```python
from build123d import *

# Parameters (mm, degrees)
SKETCH1_R           = 15
SKETCH1_R_2         = 14
BOSS_EXTRUDE1_DEPTH = 12
CUT_EXTRUDE1_DEPTH  = 31
CIRPATTERN1_COUNT   = 5
CUT_EXTRUDE2_DEPTH  = 32
CIRPATTERN2_COUNT   = 10


with BuildPart() as part:
    # Sketch1 → Boss-Extrude1 (new body)
    with BuildSketch(Plane.XY):
        Circle(SKETCH1_R)
        Circle(SKETCH1_R_2, mode=Mode.SUBTRACT)
    extrude(amount=BOSS_EXTRUDE1_DEPTH)

    # Sketch2 → Cut-Extrude1 (cut, symmetric)
    with BuildSketch(Plane(origin=(0, 0, 0), x_dir=(0, 0, -1), z_dir=(1, 0, 0))):
        Polygon((-1.5, 0), (-1.5, 3.5), (-10.5, 0), (-1.5, -3.5), align=None)
    cut_extrude1 = extrude(amount=CUT_EXTRUDE1_DEPTH, both=True, mode=Mode.SUBTRACT)

    # CirPattern1: Cut-Extrude1 ×5 about axis
    cirpattern1_axis = Axis((0, 0, 0), (0, 0, 1))
    for i in range(1, CIRPATTERN1_COUNT):
        add(cut_extrude1.rotate(cirpattern1_axis, i * 360 / CIRPATTERN1_COUNT), mode=Mode.SUBTRACT)

    # Sketch7 → Cut-Extrude2 (cut)
    with BuildSketch(Plane(origin=(-4.635254916, 14.265847744, 0), x_dir=(0.9510565162951501, 0.30901699437495833, 0), z_dir=(-0.30901699437495833, 0.9510565162951502, 0))):
        Polygon((-1.041848082, -10.5), (-4.541848082, -1.5), (-7.776778784, -10.5), align=None)
    cut_extrude2 = extrude(amount=-CUT_EXTRUDE2_DEPTH, mode=Mode.SUBTRACT)

    # CirPattern2: Cut-Extrude2 ×10 about axis
    cirpattern2_axis = Axis((0, 0, 0), (0, 0, 1))
    for i in range(1, CIRPATTERN2_COUNT):
        add(cut_extrude2.rotate(cirpattern2_axis, i * 360 / CIRPATTERN2_COUNT), mode=Mode.SUBTRACT)


solid = part.part
```
The model under review builds one solid part; all positions refer to its coordinate system, in mm. A direction names the side the tool comes from. Give positions to 0.01 mm unless a question says otherwise; leave off trailing zeros. Write each loop counter-clockwise with the first axis right and the second up, starting at its lowest first coordinate (ties: lowest second). Pieces come first, ordered by that corner, then holes. Notation, with made-up numbers: M 52,22 L 90,22 A18 ccw 90,42 Z; hole C 65,-24 d6. An arc over 180 degrees is marked long. Answer in a Markdown table with one row per item.
Item 1: Add section C-C on y = -2. Give the boundary of the cut face in (x, z), plus the area to 3 significant figures.
Check sheet entries:
| item | result |
|---|---|
| outline | M -14.87,0 L -13.86,0 L -13.86,1.5 L -14.87,1.5 Z; M -14.87,5.36 L -13.86,5.36 L -13.86,7.02 L -14.48,8.04 L -14.87,8.04 Z; M -14.87,10.5 L -13.86,10.5 L -13.86,12 L -14.87,12 Z; M 13.86,0 L 14.87,0 L 14.87,1.5 L 13.86,1.5 Z; M 13.86,5.36 L 14.87,5.36 L 14.87,8.04 L 14.48,8.04 L 13.86,7.02 Z; M 13.86,10.5 L 14.87,10.5 L 14.87,12 L 13.86,12 Z |
| area | 10.8 mm2 |
Item 2: Add section A-A on x = 7. Give the boundary of the cut face in (y, z).
Check sheet entries:
| item | result |
|---|---|
| outline | M -13.27,0 L -12.12,0 L -12.12,1.5 L -13.27,1.5 Z; M -13.27,3.92 L -12.12,3.02 L -12.12,4.71 L -12.8,6.23 L -13.27,6.6 Z; M -13.27,10.5 L -12.12,10.5 L -12.12,12 L -13.27,12 Z; M 12.12,0 L 13.27,0 L 13.27,1.5 L 12.12,1.5 Z; M 12.12,3.02 L 13.27,3.92 L 13.27,6.6 L 12.8,6.23 L 12.12,4.71 Z; M 12.12,10.5 L 13.27,10.5 L 13.27,12 L 12.12,12 Z |
Item 3: Add section B-B on z = 11. Give the boundary of the cut face in (x, y).
Check sheet entries:
| item | result |
|---|---|
| outline | C 0,0 d30; hole C 0,0 d28 |
Item 4: Add section D-D on z = 6.75. State how many separate pieces and enclosed holes the cut face has, plus the area to 3 significant figures.
Check sheet entries:
| item | result |
|---|---|
| separate pieces | 20 |
| enclosed holes | 0 |
| area | 18.7 mm2 |
Item 5: For P1, Ø1.6, axis at x = -9.5, y = -10.5, coming from the -Z side; P2, Ø1.5, axis at x = -4, z = 8.5, coming from the -Y side; P3, Ø4, axis at x = 7, z = 9.5, coming from the -Y side; P4, Ø5, axis at x = 5, z = 7, coming from the +Y side, all flat-tipped, find the tip position at first contact; note any pin that passes through.
Check sheet entries:
| item | result |
|---|---|
| P1 | z = 0 |
| P2 | y = -14.64 |
| P3 | y = -14.14 |
| P4 | y = 14.79 |
Item 6: Draft analysis for pull direction X (two halves, no side actions). For faces 3 (the face through (-10.164, 10.805, 6.063)), 4 (the face through (-6.1, 13.19, 6.06)), state which applies: +X half, -X half, draft (parallel to the pull), parting line (faces both ways), or undercut.
Check sheet entries:
| item | result |
|---|---|
| face 3 | undercut |
| face 4 | undercut |
Item 7: For line 1 along X through (y, z) = (0.5, 11); line 2 along X through (y, z) = (10.5, 4), list the stretches that pass through material, from the lowest coordinate up.
Check sheet entries:
| item | result |
|---|---|
| line 1 | -14.99 to -13.99, 13.99 to 14.99 |
| line 2 | -10.15 to -9.26, 9.26 to 10.15 |
Item 8: Tool access review of faces 1 (the face through (1.864, -14.171, 5.979)), 2 (the face through (6.822, -12.226, 4.639)): name each direction out of +Z, -Z, +X, -X, +Y, -Y from which nothing blocks a thin tool from reaching the whole face with its end or side.
Check sheet entries:
| item | result |
|---|---|
| face 1 | none |
| face 2 | +Z, -Z |
